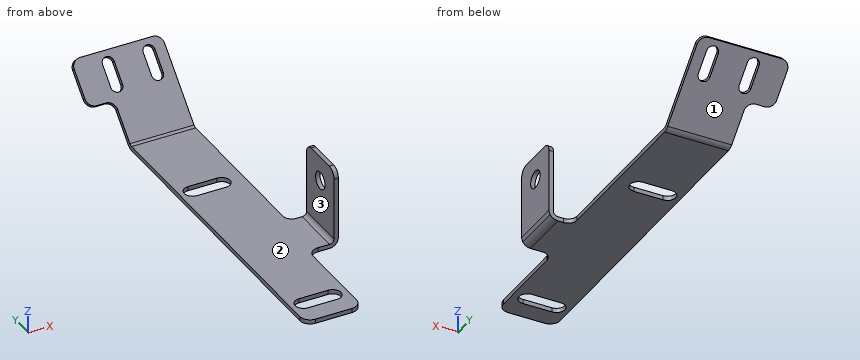
```python
from build123d import *

# Parameters (mm, degrees)
BASE_FLANGE1_DEPTH     = 3
CUT_EXTRUDE1_DEPTH     = 10
SKETCHED_START         = 179.903820644
SKETCHED_BEND1_DEPTH   = 9.096179356
SKETCHED_START_2       = -37
SKETCHED_BEND1_2_DEPTH = 62
SKETCHED_START_3       = -19
SKETCHED_BEND1_3_DEPTH = 44
SKETCHED_START_4       = -10.35
SKETCHED_BEND1_4_DEPTH = 20
SKETCHED_START_5       = -31
SKETCHED_BEND1_5_DEPTH = 12.65
SKETCHED_START_6       = 17.65
SKETCHED_BEND1_6_DEPTH = 1.35
SKETCHED_START_7       = 142.46468863
SKETCHED_BEND1_7_DEPTH = 2.999999999
SKETCHED_START_8       = 50.5
SKETCHED_BEND2_DEPTH   = 35
SKETCHED_BEND2_2_DEPTH = 35
SKETCHED_START_9       = 31
SKETCHED_BEND2_3_DEPTH = 11
SKETCH9_R              = 6
CUT_EXTRUDE2_DEPTH     = 10
CUT_EXTRUDE3_DEPTH     = 10


with BuildPart() as part:
    # Base-Flange1: sheet metal written as solids
    # Sketch1 → Base-Flange1 (new body)
    with BuildSketch(Plane(origin=(0, 0, 0), x_dir=(0, 1, 0), z_dir=(0, 0, 1))):
        with BuildLine():
            Line((-19, 12), (-19, -13))
            ThreePointArc((-19, -13), (-16.949747468, -17.949747468), (-12, -20))
            Line((-12, -20), (43.5, -20))
            ThreePointArc((43.5, -20), (48.449747468, -22.050252532), (50.5, -27))
            Line((50.5, -27), (50.5, -85))
            ThreePointArc((50.5, -85), (52.257359313, -89.242640687), (56.5, -91))
            Line((56.5, -91), (79.5, -91))
            ThreePointArc((79.5, -91), (83.742640687, -89.242640687), (85.5, -85))
            Line((85.5, -85), (85.5, -31))
            ThreePointArc((85.5, -31), (87.257359313, -26.757359313), (91.5, -25))
            Line((91.5, -25), (260, -25))
            ThreePointArc((260, -25), (264.242640687, -23.242640687), (266, -19))
            Line((266, -19), (266, 31))
            ThreePointArc((266, 31), (264.242640687, 35.242640687), (260, 37))
            Line((260, 37), (240.82, 37))
            ThreePointArc((240.82, 37), (236.577359313, 35.242640687), (234.82, 31))
            Line((234.82, 31), (234.82, 25))
            ThreePointArc((234.82, 25), (233.062640687, 20.757359313), (228.82, 19))
            Line((228.82, 19), (-12, 19))
            ThreePointArc((-12, 19), (-16.949747468, 16.949747468), (-19, 12))
        make_face()
    extrude(amount=BASE_FLANGE1_DEPTH)

    # Sketch6 → Cut-Extrude1 (cut)
    with BuildSketch(Plane.XY.offset(3)):
        with BuildLine():
            Line((9.65, 243), (9.65, 258))
            ThreePointArc((9.65, 258), (13.65, 262), (17.65, 258))
            Line((17.65, 258), (17.65, 243))
            ThreePointArc((17.65, 243), (13.65, 239), (9.65, 243))
        make_face()
        with BuildLine():
            Line((-18.35, 243), (-18.35, 258))
            ThreePointArc((-18.35, 258), (-14.35, 262), (-10.35, 258))
            Line((-10.35, 258), (-10.35, 243))
            ThreePointArc((-10.35, 243), (-14.35, 239), (-18.35, 243))
        make_face()
    extrude(amount=-CUT_EXTRUDE1_DEPTH, mode=Mode.SUBTRACT)

    # Sketched Bend1: read off the stored shape, not the designer's step
    # Sketched Bend1 outline → Sketched Bend1 (cut)
    with BuildSketch(Plane(origin=(0, 0, 0), x_dir=(1, 0, 0), z_dir=(0, 0.707106781186549, -0.707106781186546)).offset(SKETCHED_START)):
        with BuildLine():
            Line((9.65, -184.182824136), (9.65, -199.182824136))
            ThreePointArc((9.65, -199.182824136), (13.65, -203.182824136), (17.65, -199.182824136))
            Line((17.65, -199.182824136), (17.65, -184.182824136))
            ThreePointArc((17.65, -184.182824136), (13.65, -180.182824136), (9.65, -184.182824136))
        make_face()
        with BuildLine():
            Line((-18.35, -184.182824136), (-18.35, -199.182824136))
            ThreePointArc((-18.35, -199.182824136), (-14.35, -203.182824136), (-10.35, -199.182824136))
            Line((-10.35, -199.182824136), (-10.35, -184.182824136))
            ThreePointArc((-10.35, -184.182824136), (-14.35, -180.182824136), (-18.35, -184.182824136))
        make_face()
    extrude(amount=SKETCHED_BEND1_DEPTH, mode=Mode.SUBTRACT)

    # Sketched Bend1 2 outline → Sketched Bend1 2 (cut)
    with BuildSketch(Plane.YZ.offset(SKETCHED_START_2)):
        with BuildLine():
            Line((208.718135506, 3), (207.475494819, 1.757359313))
            ThreePointArc((207.475494819, 1.757359313), (205.528954726, 0.456722805), (203.232854132, 0))
            Line((203.232854132, 0), (266, 0))
            Line((266, 0), (266, 3))
            Line((266, 3), (208.718135506, 3))
        make_face()
    extrude(amount=SKETCHED_BEND1_2_DEPTH, mode=Mode.SUBTRACT)

    # Sketched Bend1 3 outline → Sketched Bend1 3 (add)
    with BuildSketch(Plane.YZ.offset(SKETCHED_START_3)):
        with BuildLine():
            Line((225.190537865, 23.715043045), (205.354174476, 3.878679656))
            ThreePointArc((205.354174476, 3.878679656), (204.380904429, 3.228361402), (203.232854132, 3))
            Line((203.232854132, 3), (208.718135506, 3))
            Line((208.718135506, 3), (227.311858208, 21.593722702))
            Line((227.311858208, 21.593722702), (225.190537865, 23.715043045))
        make_face()
    extrude(amount=SKETCHED_BEND1_3_DEPTH)

    # Sketched Bend1 4 outline → Sketched Bend1 4 (add)
    with BuildSketch(Plane.YZ.offset(SKETCHED_START_4)):
        Polygon((247.238127302, 45.762632482), (225.190537865, 23.715043045), (227.311858208, 21.593722702), (249.359447645, 43.641312139), align=None)
    extrude(amount=SKETCHED_BEND1_4_DEPTH)

    # Sketched Bend1 5 outline → Sketched Bend1 5 (add)
    with BuildSketch(Plane.YZ.offset(SKETCHED_START_5)):
        Polygon((247.238127302, 45.762632482), (225.190537865, 23.715043045), (227.311858208, 21.593722702), (249.359447645, 43.641312139), align=None)
    extrude(amount=SKETCHED_BEND1_5_DEPTH)

    # Sketched Bend1 6 outline → Sketched Bend1 6 (add)
    with BuildSketch(Plane.YZ.offset(SKETCHED_START_6)):
        Polygon((247.238127302, 45.762632482), (225.190537865, 23.715043045), (227.311858208, 21.593722702), (249.359447645, 43.641312139), align=None)
    extrude(amount=SKETCHED_BEND1_6_DEPTH)

    # Sketched Bend1 7 outline → Sketched Bend1 7 (add)
    with BuildSketch(Plane(origin=(0, 0, 0), x_dir=(1, 0, 0), z_dir=(0, 0.707106781186549, -0.707106781186546)).offset(SKETCHED_START_7)):
        with BuildLine():
            ThreePointArc((-19, -170.002824136), (-20.757359313, -174.245464823), (-25, -176.002824136))
            Line((-25, -176.002824136), (-19, -176.002824137))
            Line((-19, -176.002824137), (-19, -170.002824136))
        make_face()
        with BuildLine():
            ThreePointArc((-37, -201.182824136), (-35.242640687, -205.425464823), (-31, -207.182824136))
            Line((-31, -207.182824136), (-31, -176.002824136))
            ThreePointArc((-31, -176.002824136), (-35.242640687, -177.760183449), (-37, -182.002824136))
            Line((-37, -182.002824136), (-37, -201.182824136))
        make_face()
        with BuildLine():
            Line((-18.35, -207.182824136), (-10.35, -207.182824136))
            Line((-10.35, -207.182824136), (-10.35, -199.182824136))
            ThreePointArc((-10.35, -199.182824136), (-14.35, -203.182824136), (-18.35, -199.182824136))
            Line((-18.35, -199.182824136), (-18.35, -207.182824136))
        make_face()
        with BuildLine():
            Line((9.65, -207.182824136), (17.65, -207.182824136))
            Line((17.65, -207.182824136), (17.65, -199.182824136))
            ThreePointArc((17.65, -199.182824136), (13.65, -203.182824136), (9.65, -199.182824136))
            Line((9.65, -199.182824136), (9.65, -207.182824136))
        make_face()
        with BuildLine():
            Line((25, -201.182824136), (25, -176.002824137))
            Line((25, -176.002824137), (19, -176.002824137))
            Line((19, -176.002824137), (19, -207.182824136))
            ThreePointArc((19, -207.182824136), (23.242640687, -205.425464823), (25, -201.182824136))
        make_face()
        with BuildLine():
            ThreePointArc((9.65, -184.182824136), (13.65, -180.182824136), (17.65, -184.182824136))
            Line((17.65, -184.182824136), (17.65, -176.002824137))
            Line((17.65, -176.002824137), (9.65, -176.002824137))
            Line((9.65, -176.002824137), (9.65, -184.182824136))
        make_face()
        with BuildLine():
            ThreePointArc((-18.35, -184.182824136), (-14.35, -180.182824136), (-10.35, -184.182824136))
            Line((-10.35, -184.182824136), (-10.35, -176.002824137))
            Line((-10.35, -176.002824137), (-18.35, -176.002824137))
            Line((-18.35, -176.002824137), (-18.35, -184.182824136))
        make_face()
    extrude(amount=SKETCHED_BEND1_7_DEPTH)

    # Sketched Bend2: read off the stored shape, not the designer's step
    # Sketched Bend2 outline → Sketched Bend2 (cut)
    with BuildSketch(Plane(origin=(0, 0, 0), x_dir=(1, 0, 0), z_dir=(0, 1, 0)).offset(SKETCHED_START_8)):
        with BuildLine():
            ThreePointArc((35, 0), (38, -0.803847577), (40.196152423, -3))
            Line((40.196152423, -3), (91, -3))
            Line((91, -3), (91, 0))
            Line((91, 0), (35, 0))
        make_face()
    extrude(amount=SKETCHED_BEND2_DEPTH, mode=Mode.SUBTRACT)

    # Sketched Bend2 2 outline → Sketched Bend2 2 (add)
    with BuildSketch(Plane(origin=(0, 0, 0), x_dir=(1, 0, 0), z_dir=(0, 1, 0)).offset(SKETCHED_START_8)):
        with BuildLine():
            ThreePointArc((35, -3), (37.121320344, -3.878679656), (38, -6))
            Line((38, -6), (38, -54.931416529))
            Line((38, -54.931416529), (41, -54.931416529))
            Line((41, -54.931416529), (41, -6))
            ThreePointArc((41, -6), (40.795554958, -4.447085729), (40.196152423, -3))
            Line((40.196152423, -3), (35, -3))
        make_face()
    extrude(amount=SKETCHED_BEND2_2_DEPTH)

    # Sketched Bend2 3 outline → Sketched Bend2 3 (cut)
    with BuildSketch(Plane.YZ.offset(SKETCHED_START_9)):
        with BuildLine():
            ThreePointArc((50.5, 48.931416529), (52.257359313, 53.174057216), (56.5, 54.931416529))
            Line((56.5, 54.931416529), (50.5, 54.931416529))
            Line((50.5, 54.931416529), (50.5, 48.931416529))
        make_face()
        with BuildLine():
            ThreePointArc((79.5, 54.931416529), (83.742640687, 53.174057217), (85.5, 48.931416529))
            Line((85.5, 48.931416529), (85.5, 54.931416529))
            Line((85.5, 54.931416529), (79.5, 54.931416529))
        make_face()
    extrude(amount=SKETCHED_BEND2_3_DEPTH, mode=Mode.SUBTRACT)

    # Sketch9 → Cut-Extrude2 (cut)
    with BuildSketch(Plane.YZ.offset(41)):
        with Locations(Location((68, 38, 0), (0, 0, 270))):
            Circle(SKETCH9_R)
    extrude(amount=-CUT_EXTRUDE2_DEPTH, mode=Mode.SUBTRACT)

    # Sketch10 → Cut-Extrude3 (cut)
    with BuildSketch(Plane.XY.offset(3)):
        with BuildLine():
            Line((-10, 5.75), (10, 5.75))
            ThreePointArc((10, 5.75), (15.75, 0), (10, -5.75))
            Line((10, -5.75), (-10, -5.75))
            ThreePointArc((-10, -5.75), (-15.75, 0), (-10, 5.75))
        make_face()
        with BuildLine():
            Line((-10, 147.75), (10, 147.75))
            ThreePointArc((10, 147.75), (15.75, 142), (10, 136.25))
            Line((10, 136.25), (-10, 136.25))
            ThreePointArc((-10, 136.25), (-15.75, 142), (-10, 147.75))
        make_face()
    extrude(amount=-CUT_EXTRUDE3_DEPTH, mode=Mode.SUBTRACT)


solid = part.part
```
Model file for the job. Use its own axes, mm. Face numbers are marked on the shaded views. A direction names the side the tool comes from. Give positions to 0.01 mm unless a question says otherwise; leave off trailing zeros. Order: outer loops, then holes, each group sorted by start corner. A loop starts at its lowest first (then second) coordinate and runs counter-clockwise, first axis right, second up.
1) Wall check: probe 1 along Y at (x, z) = (39.9, 38); probe 2 along Z at (x, y) = (10, 44); probe 3 along X at (y, z) = (70, 6). Give the ranges that are in metal, low to high.
2) Saw through at C-C, the plane y = 172. Write the cut outline in (x, z), then the cut area to 3 significant figures.
3) 3-axis set-ups, long thin cutter, end or side, ignore diameter. For the marked faces 1, 2 and 3: which of +Z, -Z, +X, -X, +Y, -Y reach the whole face in a straight line?
4) Saw through at B-B, the plane y = 68. Write the cut outline in (x, z).
5) Pin check, flat tips, straight feed: pin 1 (5 mm diameter, centred on x = -2.5, z = 26, fed in from -Y); pin 2 (5 mm diameter, centred on x = -7, y = 218.5, fed in from -Z); pin 3 (17.5 mm diameter, centred on y = 64, z = 21.5, fed in from -X). Stop position of each tip, or through.
6) Saw through at A-A, the plane y = 142. Write the cut outline in (x, z).
Computed:
1. probe 1: y = 50.5 to 62, 74 to 85.5
1. probe 2: z = 0 to 3
1. probe 3: x = 38 to 41
2. outline: (-19, 0) - (25, 0) - (25, 3) - (-19, 3) - close
2. area: 132 mm2
3. face 1: -Z, +X, -X, +Y
3. face 2: +Z, -X, -Y
3. face 3: +Z, -X, +Y, -Y
4. outline: (-19, 0) - (35, 0) arc R6 ccw to (41, 6) - (41, 32) - (38, 32) - (38, 6) arc R3 cw to (35, 3) - (-19, 3) - close; (38, 44) - (41, 44) - (41, 54.93) - (38, 54.93) - close
5. pin 1: stops at y = 224.98
5. pin 2: stops at z = 10.28
5. pin 3: stops at x = 38
6. outline: (-19, 0) - (-15.75, 0) - (-15.75, 3) - (-19, 3) - close; (15.75, 0) - (25, 0) - (25, 3) - (15.75, 3) - close
